Work out the finished part from the listing and answer in its coordinate system (mm). A direction names the side the tool comes from. Coordinates: 2 decimals unless noted, no trailing zeros. Order: outer loops, then holes, each group sorted by start corner. A loop starts at its lowest first (then second) coordinate and runs counter-clockwise, first axis right, second up. Notation, with made-up numbers: M 75,29.5 L 100,29.5 A25 cw 100,51.5 Z; hole C 38,-20.75 d2. An arc over 180 degrees is marked long. Answer in a Markdown table with one row per item. Add a question column.
Item 1: Which of the six approach directions +Z, -Z, +X, -X, +Y, -Y give full straight-line access (tool end or side, diameter ignored) to faces 1 (the face through (-30, 2, -110)), 2 (the face through (-56, 5, -59)), 3 (the face through (-143, 3, -10)), 4 (the face through (-149.958, 21.712, -118.147))?
Item 2: The part is cut by section D-D (z = -115). Write down the section's boundary in (x, y), then the cut area to 3 significant figures.
Item 3: Flat-ended cylindrical pins translate along their axes: pin 1 Ø7 at (y, z) = (20.5, -114) entering from +X; pin 2 Ø3.5 at (x, z) = (-108, -15) entering from +Y; pin 3 Ø4 at (y, z) = (2, -72) entering from -X; pin 4 Ø8 at (x, y) = (-88.5, 12) entering from -Z. Find the tip coordinate at first contact, or state that the pin passes through.
Item 4: The part is cut by section A-A (x = -143.5). Write down the section's boundary in (y, z).
Item 5: The mould has two halves that part along Y. Classify faces 5 (the face through (-113, 2, -61)), 6 (the face through (-153, 22, -115)), 7 (the face through (-151.06, 26.85, -114.89)): released by +Y, released by -Y, zero draft, split by the parting line, or undercut.
Item 6: Consider line 1 (X direction, y = 2.9, z = -15); line 2 (Z direction, x = -108, y = 3.65); line 3 (X direction, y = 1.75, z = -32.5). Determine where each line is inside the solid, lowest interval first. Write a range as from..to.
Item 7: The part is cut by section B-B (z = -79.5). Write down the section's boundary in (x, y).
Item 8: The part is cut by section C-C (y = 8.75). Write down the section's boundary in (x, z), then the cut area to 3 significant figures.
Autodesk Inventor part; units mm, degrees
ref_plane "Work Plane1" through (-155, 0, -60) normal (0, 0, 1) x (1, 0, 0)
ref_plane "YZ Plane" through (0, 0, 0) normal (1, 0, 0) x (0, 1, 0)
ref_plane "XZ Plane" through (0, 0, 0) normal (0, 1, 0) x (-1, 0, 0)
sketch "Sketch1" plane through (0, 0, 0) normal (0, 1, 0) x (-1, 0, 0)
  line L0 (0, 0) -> (0, -120)
  line L1 (0, -120) -> (155, -120)
  line L2 (155, -120) -> (155, -110)
  line L3 (155, -110) -> (113, -110)
  line L4 (113, -110) -> (113, -10)
  line L5 (113, -10) -> (155, -10)
  line L6 (155, -10) -> (155, 0)
  line L7 (155, 0) -> (0, 0)
  line L8 (103, -10) -> (61.5, -10)
  line L9 (61.5, -10) -> (61.5, -110)
  line L10 (61.5, -110) -> (103, -110)
  line L11 (103, -110) -> (103, -10)
  line L12 (51.5, -10) -> (10, -10)
  line L13 (10, -10) -> (10, -110)
  line L14 (10, -110) -> (51.5, -110)
  line L15 (51.5, -110) -> (51.5, -10)
  dimension "d1" = 155
  dimension "d2" = 10
  dimension "d3" = 120
  dimension "d4" = 10
  dimension "d5" = 10
  dimension "d6" = 10
  dimension "d16" = 41.5
extrude "Extrusion1" add sketch "Sketch1" along normal blind 5
sketch "Sketch2" plane through (-155, 0, -10) normal (-1, 0, 0) x (0, 0, 1)
  line L0 (0, 0) -> (0, 5)
  line L1 (0, 0) -> (10, 0)
  line L2 (10, 0) -> (10, 21.85)
  line L3 (10, 21.85) -> (0, 21.85)
  line L4 (0, 21.85) -> (0, 0)
  circle A0 centre (5, 21.85) radius 3.15
  arc A1 (10, 21.85) -> (0, 21.85) centre (5, 21.85) ccw
  line L5 (10, 0) -> (10, 5)
  point P0 (0, 5)
  dimension "d9" = 21.85
  dimension "d10" = 6.3
extrude "Extrusion2" add sketch "Sketch2" against normal blind 8
sketch "Sketch3" plane through (-147, 0, -10) normal (1, 0, 0) x (0, 0, -1)
  arc A0 (0, 21.85) -> (-10, 21.85) centre (-5, 21.85) ccw
  circle A1 centre (-5, 21.85) radius 3.15
  point P0 (-10, 0)
  dimension "d13" = 6.3
extrude "Extrusion3" cut sketch "Sketch3" against normal blind 6
ref_plane "Work Plane1" through (-155, 0, -60) normal (0, 0, 1) x (1, 0, 0)
mirror "Mirror1" about plane through (-155, 0, -60) normal (0, 0, 1) of "Extrusion2", "Extrusion3"
sketch "Sketch4" plane through (0, 5, 0) normal (0, 1, 0) x (1, 0, 0)
  line L0 (-113, 110) -> (-113, 10)
  line L1 (-147, 0) -> (0, 0)
  point P0 (-108, 15)
  point P1 (-56.5, 15)
  point P2 (-108, 105)
  point P3 (-56.5, 105)
  dimension "d17" = 5
  dimension "d18" = 15
  dimension "d21" = 51.5
  dimension "d24" = 90
hole "Hole1" at (-108, 5, -15) at (-56.5, 5, -15) at (-108, 5, -105) at (-56.5, 5, -105) direction (0, -1, 0) diameter 3 end through all
equation "\"d1\" = table_base_length"
equation "\"d2\" = table_base_web_width"
equation "\"d3\" = table_base_width"
equation "\"d4\" = table_base_web_width"
equation "\"d5\" = table_base_web_width"
equation "\"d6\" = table_base_web_width"
equation "\"d7\" = table_base_thickness"
equation "\"d10\" = rod_diameter + rod_tolerance"
equation "\"d11\" = table_base_rod_holder_thickness"
equation "\"d13\" = rod_diameter + rod_tolerance"
equation "\"d14\" = 0.75 * table_base_rod_holder_thickness"
equation "\"d27\" = screw_diameter"
equation "\"table_base_length\" = 155"
equation "\"table_base_width\" = 120"
equation "\"table_base_thickness\" = 5"
equation "\"table_base_web_width\" = 10"
equation "\"table_base_rod_height\" = 25"
equation "\"rod_diameter\" = 6"
equation "\"rod_tolerance\" = 0.3"
equation "\"table_base_rod_holder_thickness\" = 8"
equation "\"screw_diameter\" = 3"
properties part number "table_base"
Reply:
| question | item | result |
|---|---|---|
| 1 | face 1 | +Y, -Y |
| 1 | face 2 | +Z, -Z, +X, +Y |
| 1 | face 3 | -X, +Y, -Y |
| 1 | face 4 | +X |
| 2 | outline | M -155,0 L 0,0 L 0,5 L -147,5 L -147,18.7 L -153,18.7 L -153,25 L -147,25 L -147,26.85 L -155,26.85 Z |
| 2 | area | 912 mm2 |
| 3 | pin 1 | stops at x = -147 |
| 3 | pin 2 | stops at y = 5 |
| 3 | pin 3 | stops at x = -113 |
| 3 | pin 4 | passes through |
| 4 | outline | M 0,-120 L 5,-120 L 5,-110 L 0,-110 Z; M 0,-10 L 5,-10 L 5,0 L 0,0 Z |
| 5 | face 5 | zero draft |
| 5 | face 6 | undercut |
| 5 | face 7 | released by +Y |
| 6 | line 1 | x = -113..-109.5, -106.5..-103, -61.5..-58, -55..-51.5, -10..0 |
| 6 | line 2 | z = -120..-106.5, -103.5..-16.5, -13.5..0 |
| 6 | line 3 | x = -113..-103, -61.5..-51.5, -10..0 |
| 7 | outline | M -113,0 L -103,0 L -103,5 L -113,5 Z; M -61.5,0 L -51.5,0 L -51.5,5 L -61.5,5 Z; M -10,0 L 0,0 L 0,5 L -10,5 Z |
| 8 | outline | M -155,-120 L -147,-120 L -147,-110 L -155,-110 Z; M -155,-10 L -147,-10 L -147,0 L -155,0 Z |
| 8 | area | 160 mm2 |
